from build123d import *
from build123d.topology import SkipClean

# Parameters (mm, degrees)
SKETCH1_R           = 1.2
BOSS_EXTRUDE1_DEPTH = 2
BOSS_EXTRUDE2_START = 3.2
SKETCH2_R           = 1.2
BOSS_EXTRUDE2_DEPTH = 3.2
SKETCH3_R           = 2.4
CUT_EXTRUDE3_DEPTH  = 3.2
SKETCH4_R           = 2.75
CUT_EXTRUDE4_DEPTH  = 1


with BuildPart() as part:
    # Sketch1 → Boss-Extrude1 (new body)
    with BuildSketch(Plane(origin=(0, 0, 0), x_dir=(1, 0, 0), z_dir=(0, 1, 0))):
        with BuildLine():
            Line((0.356514085, 3.73301456), (14.428169014, 2.389129319))
            ThreePointArc((14.428169014, 2.389129319), (16.6, 0), (14.428169014, -2.389129319))
            Line((14.428169014, -2.389129319), (0.356514085, -3.73301456))
            ThreePointArc((0.356514085, -3.73301456), (-3.75, 0), (0.356514085, 3.73301456))
        make_face()
        with Locations(Location((0, 0, 0), (0, 0, 270))):
            Circle(SKETCH1_R, mode=Mode.SUBTRACT)
    extrude(amount=BOSS_EXTRUDE1_DEPTH)

    # Sketch2 → Boss-Extrude2 (add)
    with SkipClean():  # the faces are left unmerged after this step: merging them gives an invalid solid
        with BuildSketch(Plane.XZ.offset(BOSS_EXTRUDE2_START)):
            with BuildLine():
                ThreePointArc((3.75, 0), (2.774835835, 2.522456361), (0.356514085, 3.73301456))
                ThreePointArc((0.356514085, 3.73301456), (-3.75, 0), (0.356514085, -3.73301456))
                ThreePointArc((0.356514085, -3.73301456), (2.774835835, -2.522456361), (3.75, 0))
            make_face()
            with Locations(Location((0, 0, 0), (0, 0, 270))):
                Circle(SKETCH2_R, mode=Mode.SUBTRACT)
        extrude(amount=-BOSS_EXTRUDE2_DEPTH)

    # Sketch3 → Cut-Extrude3 (cut)
    with BuildSketch(Plane.XZ.offset(3.2)):
        with Locations(Location((0, 0, 0), (0, 0, 270))):
            Circle(SKETCH3_R)
    extrude(amount=-CUT_EXTRUDE3_DEPTH, mode=Mode.SUBTRACT)

    # Sketch4 → Cut-Extrude4 (cut)
    with BuildSketch(Plane(origin=(0, 2, 0), x_dir=(1, 0, 0), z_dir=(0, 1, 0))):
        with Locations(Location((0, 0, 0), (0, 0, 270))):
            Circle(SKETCH4_R)
    extrude(amount=-CUT_EXTRUDE4_DEPTH, mode=Mode.SUBTRACT)


solid = part.part
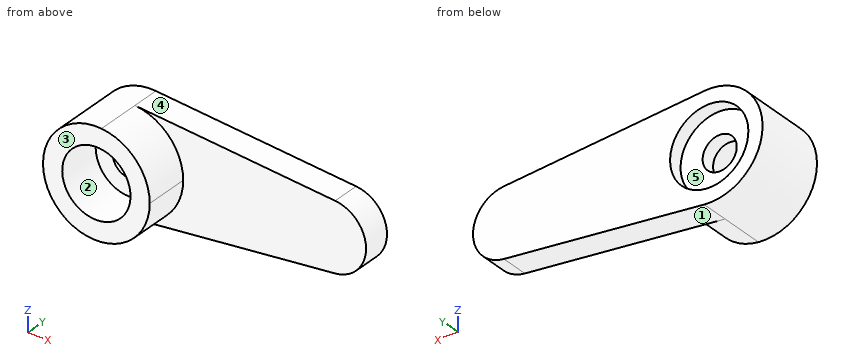
Build history of the part. All positions in model axes, mm. Face numbers are marked on the shaded views. A direction names the side the tool comes from. Give positions to 0.01 mm unless a question says otherwise; leave off trailing zeros. Order: outer loops, then holes, each group sorted by start corner. A loop starts at its lowest first (then second) coordinate and runs counter-clockwise, first axis right, second up. Notation, with made-up numbers: M 33.5,23 L 64.5,23 A10 cw 64.5,37 Z; hole C -2,64.5 d5. An arc over 180 degrees is marked long. Put each result on its own line as item: value.
Item 1: Cut at C-C on z = -1.5. Write the cut outline in (x, y), then the cut area to 3 significant figures.
Results are:
outline: M -3.44,-3.2 L -1.87,-3.2 L -1.87,0 L 1.87,0 L 1.87,-3.2 L 3.44,-3.2 L 3.44,0 L 16.07,0 L 16.07,2 L 2.3,2 L 2.3,1 L -2.3,1 L -2.3,2 L -3.44,2 Z
area: 44.4 mm2
Item 2: Pull direction X, two halves, no side cores. Call the marked faces 1, 2 and 3: +X half, -X half, draft (parallel to the pull), parting line (faces both ways), or undercut.
Results are:
face 1: +X half
face 2: undercut
face 3: draft
Item 3: Cut at B-B on y = 1.5. Write the cut outline in (x, z).
Results are:
outline: M 0.36,-3.73 L 14.43,-2.39 A2.4 ccw 14.43,2.39 L 0.36,3.73 A3.75 ccw long Z; hole C 0,0 d5.5
Item 4: Drop flat-ended pins along their axis: pin 1 Ø1.6 at (x, z) = (-0.5, 1) entering from +Y; pin 2 Ø2 at (x, z) = (14.5, 1.5) entering from -Y. Give the stop position or say it passes through.
Results are:
pin 1: y = 1
pin 2: y = 0
Item 5: Cut at D-D on z = -0.5. Write the cut outline in (x, y), then the cut area to 3 significant figures.
Results are:
outline: M -3.72,-3.2 L -2.35,-3.2 L -2.35,0 L -1.09,0 L -1.09,1 L -2.7,1 L -2.7,2 L -3.72,2 Z; M 1.09,0 L 2.35,0 L 2.35,-3.2 L 3.72,-3.2 L 3.72,0 L 16.55,0 L 16.55,2 L 2.7,2 L 2.7,1 L 1.09,1 Z
area: 41.7 mm2
Item 6: Which spindle directions (+Z, -Z, +X, -X, +Y, -Y) get a long thin tool onto all of the face, cutting with end or side? Do the marked faces 4 and 5. Say none if no direction does.
Results are:
face 4: +Z, +X, +Y, -Y
face 5: +Y
Item 7: Wall check: probe 1 along X at (y, z) = (1.35, 0); probe 2 along Z at (x, y) = (0, 0.2); probe 3 along Y at (x, z) = (7.25, -1.25). Give the ranges that are in metal, low to high.
Results are:
probe 1: -3.75 to -2.75, 2.75 to 16.6
probe 2: -3.75 to -1.2, 1.2 to 3.75
probe 3: 0 to 2
Item 8: Cut at A-A on x = 0. Write the cut outline in (y, z).
Results are:
outline: M -3.2,-3.75 L 2,-3.75 L 2,-2.75 L 1,-2.75 L 1,-1.2 L 0,-1.2 L 0,-2.4 L -3.2,-2.4 Z; M -3.2,2.4 L 0,2.4 L 0,1.2 L 1,1.2 L 1,2.75 L 2,2.75 L 2,3.75 L -3.2,3.75 Z
